Work out the finished part from the listing and answer in its coordinate system (mm). A direction names the side the tool comes from. Give positions to 0.01 mm unless a question says otherwise; leave off trailing zeros. Loops run counter-clockwise (first coordinate to the right, second up) from the corner with the lowest first, then second, coordinate; pieces in that order, holes last. Notation, with made-up numbers: (-37, -28.75) - (-14, -28.75) arc R11 ccw to (-14, -10.75) - close; hole circle Ø4 at (-25.5, 1.5). An arc over 180 degrees is marked (long way). Use CSV: the item, a comma, the result in double quotes.
from build123d import *

# Parameters (mm, degrees)
EXTRUDE_1_DEPTH     = 220
SKETCH_2_R          = 3.3
CUT_EXTRUDE_1_DEPTH = 222.020361053


with BuildPart() as part:
    # Эскиз1 → Бобышка-Вытянуть1 (new body)
    with BuildSketch(Plane(origin=(0, 0, 0), x_dir=(1, 0, 0), z_dir=(0, 1, 0))):
        with BuildLine():
            Line((-7.5, 7.5), (7.5, 7.5))
            ThreePointArc((7.5, 7.5), (15, 0), (7.5, -7.5))
            Line((7.5, -7.5), (-7.5, -7.5))
            ThreePointArc((-7.5, -7.5), (-15, 0), (-7.5, 7.5))
        make_face()
        with BuildLine():
            Line((-7.5, 6), (7.5, 6))
            ThreePointArc((7.5, 6), (13.5, 0), (7.5, -6))
            Line((7.5, -6), (-7.5, -6))
            ThreePointArc((-7.5, -6), (-13.5, 0), (-7.5, 6))
        make_face(mode=Mode.SUBTRACT)
    extrude(amount=EXTRUDE_1_DEPTH)

    # Эскиз2 → Вырез-Вытянуть1 (cut, through all)
    with BuildSketch(Plane.XY.offset(7.5)):
        with Locations((0, 180)):
            Circle(SKETCH_2_R)
        with Locations((0, 140)):
            Circle(SKETCH_2_R)
        with Locations((0, 100)):
            Circle(SKETCH_2_R)
        with Locations((0, 60)):
            Circle(SKETCH_2_R)
        with Locations((0, 20)):
            Circle(SKETCH_2_R)
        Polygon((15, 220), (-15, 220), (-15, 214.710190579), align=None)
    extrude(amount=-CUT_EXTRUDE_1_DEPTH, mode=Mode.SUBTRACT)


solid = part.part
Item 1: A cutting plane is placed at D-D on z = 0. Determine the outline of the cut face in (x, y).
Determined:
outline,"(-15, 0) - (-13.5, 0) - (-13.5, 214.97) - (-15, 214.71) - close; (13.5, 0) - (15, 0) - (15, 220) - (13.5, 219.74) - close"
Item 2: For faces 1 (the cylindrical face through (1.774, 102.783, 6.76)), 2 (the cylindrical face through (13.5, 108.3, -0.1)), determine the directions among +Z, -Z, +X, -X, +Y, -Y from which every point of the face is accessible in a straight line to the end or side of a thin tool.
Determined:
face 1,"+Z, -Z"
face 2,"+Y, -Y"
Item 3: A cutting plane is placed at C-C on x = 11.5. Determine the outline of the cut face in (y, z), and give its area (3 significant figures).
Determined:
outline,"(0, -6.34) - (219.38, -6.34) - (219.38, -4.47) - (0, -4.47) - close; (0, 4.47) - (219.38, 4.47) - (219.38, 6.34) - (0, 6.34) - close"
area,"821 mm²"
Item 4: Find the intervals of material crossed by line 1 (Y direction, x = 0, z = 6.4); line 2 (Z direction, x = 7, y = 196); line 3 (X direction, y = 43, z = 0.75), in increasing order.
Determined:
line 1,"y = 0 to 16.7, 23.3 to 56.7, 63.3 to 96.7, 103.3 to 136.7, 143.3 to 176.7, 183.3 to 217.36"
line 2,"z = -7.5 to -6, 6 to 7.5"
line 3,"x = -14.96 to -13.45, 13.45 to 14.96"
Item 5: A cutting plane is placed at A-A on y = 140. Determine the outline of the cut face in (x, z), and give its area (3 significant figures).
Determined:
outline,"(-7.5, -7.5) - (-3.3, -7.5) - (-3.3, -6) - (-7.5, -6) arc R6 cw to (-7.5, 6) - (-3.3, 6) - (-3.3, 7.5) - (-7.5, 7.5) arc R7.5 ccw to start; (3.3, -7.5) - (7.5, -7.5) arc R7.5 ccw to (7.5, 7.5) - (3.3, 7.5) - (3.3, 6) - (7.5, 6) arc R6 cw to (7.5, -6) - (3.3, -6) - close"
area,"88.8 mm²"
Item 6: The mould has two halves that part along X. Classify faces 3 (the cylindrical face through (15, 108, 0)), 4 (the flat face through (0, 108, 6)), 5 (the cylindrical face through (-0.72, 16.78, 6.76)), 6 (the flat face through (1.04, 217.54, 6.15)): pulls with the +X half, pulls with the -X half, needs draft (parallel to the pull), parting line crosses it, or undercut.
Determined:
face 3,"pulls with the +X half"
face 4,"undercut"
face 5,"undercut"
face 6,"pulls with the -X half"
Item 7: Given P1, Ø2, axis at x = 11.5, y = 64, coming from the +Z side; P2, Ø5, axis at y = 160, z = -3.5, coming from the +X side; P3, Ø3, axis at y = 196, z = 4.5, coming from the +X side, each flat-ended and moving along its own axis, determine where each tip first touches the part or whether it passes through.
Determined:
P1,"stops at z = 6.87"
P2,"stops at x = 14.93"
P3,"stops at x = 14.37"
Item 8: A cutting plane is placed at B-B on y = 30. Determine the outline of the cut face in (x, z), and give its area (3 significant figures).
Determined:
outline,"(-7.5, -7.5) - (7.5, -7.5) arc R7.5 ccw to (7.5, 7.5) - (-7.5, 7.5) arc R7.5 ccw to start; hole (-7.5, -6) - (7.5, -6) arc R6 ccw to (7.5, 6) - (-7.5, 6) arc R6 ccw to start"
area,"109 mm²"
